The listing builds one solid part. Answer for the finished solid, in the listing's coordinates (mm). A direction names the side the tool comes from. Give positions to 0.01 mm unless a question says otherwise; leave off trailing zeros. Write each loop counter-clockwise with the first axis right and the second up, starting at its lowest first coordinate (ties: lowest second). Pieces come first, ordered by that corner, then holes.
```python
from build123d import *

# Parameters (mm, degrees)
BOSS_EXTRUDE1_DEPTH = 11.557
FILLET1_R           = 2.54
FILLET2_R           = 0.635
SHELL1_T            = -1.016
SKETCH3_W           = 12.065
SKETCH3_H           = 1.016
BOSS_EXTRUDE2_DEPTH = 3.175
SKETCH4_R           = 1.524
SKETCH4_W           = 3.937
SKETCH4_H           = 6.477
CUT_EXTRUDE1_DEPTH  = 158.908914941
SKETCH5_R           = 2.0574
CUT_EXTRUDE2_DEPTH  = 160.727285329


with BuildPart() as part:
    # Sketch1 → Boss-Extrude1 (new, symmetric)
    with BuildSketch(Plane.XY):
        with BuildLine():
            Line((0, 0), (60.96, 0))
            Line((60.96, 0), (60.96, 2.641614405))
            ThreePointArc((60.96, 2.641614405), (62.769867337, 7.571802884), (67.339726625, 10.16))
            ThreePointArc((67.339726625, 10.16), (109.560204459, 14.953353711), (152.048769719, 15.469890784))
            ThreePointArc((152.048769719, 15.469890784), (154.303696185, 16.667899597), (154.378077788, 19.220229093))
            Line((154.378077788, 19.220229093), (147.366478068, 32.131))
            Line((147.366478068, 32.131), (4.991923978, 19.304))
            Line((4.991923978, 19.304), (0, 0))
        make_face()
    extrude(amount=BOSS_EXTRUDE1_DEPTH, both=True)

    # Fillet1
    fillet1_edges = [part.edges().sort_by_distance(p)[0] for p in [
        (76.179201023, 25.7175, 11.557),
        (76.179201023, 25.7175, -11.557),
    ]]
    fillet(fillet1_edges, radius=FILLET1_R)

    # Fillet2
    fillet2_edges = [part.edges().sort_by_distance(p)[0] for p in [
        (0, 0, 0),
    ]]
    fillet(fillet2_edges, radius=FILLET2_R)

    # Shell1
    shell1_openings = [part.faces().sort_by_distance(p)[0] for p in [
        (150.901052558, 25.62263054, 0),
        (154.303696185, 16.667899597, 0),
        (109.560204459, 14.953353711, 0),
        (62.769867337, 7.571802884, 0),
        (60.96, 1.320807203, 0),
        (30.890048092, 0, 0),
        (2.583601555, 9.990906242, 0),
        (0.318012361, 0.246236787, 0),
    ]]
    offset(amount=SHELL1_T, openings=shell1_openings, kind=Kind.INTERSECTION)

    # Sketch3 → Boss-Extrude2 (add)
    with BuildSketch(Plane(origin=(149.051444963, 13.428543441, 0), x_dir=(0, 0, -1), z_dir=(0.9959661345298199, 0.08972992181947408, 0))):
        with Locations((0, 18.270205313)):
            Rectangle(SKETCH3_W, SKETCH3_H)
    extrude(amount=BOSS_EXTRUDE2_DEPTH)

    # Sketch4 → Cut-Extrude1 (cut, through all)
    with BuildSketch(Plane(origin=(-1.684966895, 18.702456559, 0), x_dir=(0.9959661345298199, 0.08972992181947409, 0), z_dir=(-0.08972992181947409, 0.9959661345298199, 0))):
        with Locations(Location((121.969133639, 0, 0), (0, 0, 180))):
            Circle(SKETCH4_R)
        with Locations(Location((141.908133639, 0, 0), (0, 0, 180))):
            Circle(SKETCH4_R)
        with Locations((19.340433639, 0)):
            Rectangle(SKETCH4_W, SKETCH4_H)
        with Locations((133.843633639, 0)):
            Rectangle(SKETCH4_W, SKETCH4_H)
    extrude(amount=-CUT_EXTRUDE1_DEPTH, mode=Mode.SUBTRACT)

    # Sketch5 → Cut-Extrude2 (cut, through all)
    with BuildSketch(Plane.XY.offset(11.557)):
        with Locations((5.012495837, 4.064)):
            Circle(SKETCH5_R)
    extrude(amount=-CUT_EXTRUDE2_DEPTH, mode=Mode.SUBTRACT)


solid = part.part
```
Item 1: A cutting plane is placed at B-B, the plane z = 4.75. Give the vertices of the cut face in (x, y).
Conclusion:
outline: (4.72, 18.26) - (150.62, 31.4) - (150.53, 32.42) - (4.99, 19.3) - close
Item 2: Each of these flat-tipped pins is pushed along its axis until it touches: P1, Ø10, axis at x = 67, z = -9, coming from the -Y side; P2, Ø1.4, axis at x = 148.5, y = 32, coming from the +Z side; P3, Ø1.1, axis at x = 132.5, y = 30, coming from the +Z side. Where does it stop, or does it pass through?
Conclusion:
P1: stops at y = 6.87
P2: stops at z = 6.03
P3: stops at z = 11.25
Item 3: Which of the six approach directions +Z, -Z, +X, -X, +Y, -Y give full straight-line access (tool end or side, diameter ignored) to faces 1 (the face through (108.966, 14.916, 11.056)), 2 (the face through (150.1, 27.1, 10.9)), 3 (the face through (75.39, 24.19, 10.08)), 4 (the face through (76, 15, -11.557)), 5 (the face through (150.1, 27.1, -10.8))?
Conclusion:
face 1: +Z, -Z, -Y
face 2: +Z, +X, +Y
face 3: +X, -Y
face 4: -Z, +X, -X, +Y, -Y
face 5: -Z, +X, +Y
Item 4: Determine the mould class of faces 6 (the face through (154.284, 16.636, -11.042)), 7 (the face through (141.212, 31.074, 0.067)), 8 (the face through (75.328, 24.914, 10.793)), 9 (the face through (75.328, 24.914, -10.793)) for opening direction Z: pulls with the +Z half, pulls with the -Z half, needs draft (parallel to the pull), parting line crosses it, or undercut.
Conclusion:
face 6: needs draft
face 7: undercut
face 8: pulls with the +Z half
face 9: pulls with the -Z half
Item 5: A cutting plane is placed at A-A, the plane y = 13. Give the vertices of the cut face in (x, z).
Conclusion:
outline: (3.36, -11.56) - (87.61, -11.56) - (87.61, -10.54) - (3.36, -10.54) - close; (3.36, 10.54) - (87.61, 10.54) - (87.61, 11.56) - (3.36, 11.56) - close
Item 6: Consider probe 1 along Z at (x, y) = (56, 16); probe 2 along Y at (x, z) = (82, 2.75); probe 3 along Y at (x, z) = (143, -5.75). Determine where each line is inside the solid, lowest interval first.
Conclusion:
probe 1: z = -11.56 to -10.54, 10.54 to 11.56
probe 2: y = 25.22 to 26.24
probe 3: y = 30.72 to 31.74
